Work out the finished part from the listing and answer in its coordinate system (mm). A direction names the side the tool comes from. Give positions to 0.01 mm unless a question says otherwise; leave off trailing zeros. Write each loop counter-clockwise with the first axis right and the second up, starting at its lowest first coordinate (ties: lowest second). Pieces come first, ordered by that corner, then holes.
1) Straight lines are drawn through the part: probe 1 along X at (y, z) = (0.95, 32); probe 2 along Z at (x, y) = (21.5, 0.85). For each, find the intervals that lie inside material, in ascending order.
2) Determine the mould class of faces 6 (the face through (-23, 2, -31)), 7 (the face through (-20, 2, -34)), 8 (the face through (25, 2, 0)) for opening direction X: pulls with the +X half, pulls with the -X half, needs draft (parallel to the pull), parting line crosses it, or undercut.
3) Given pin 1 Ø2.5 at (x, y) = (22, 3.5) entering from +Z; pin 2 Ø2.5 at (y, z) = (3, -32.5) entering from +X, each flat-ended and moving along its own axis, determine where each tip first touches the part or whether it passes through.
4) Find section A-A (y = 2.7). Determine the outline of the cut face in (x, z).
5) A tool of negligible diameter and unlimited length cuts with its end or side. For faces 1 (the face through (0, 2, -36)), 2 (the face through (22, 2, -31)), 3 (the face through (-22, 2, 31)), 4 (the face through (23, 2, 31)), 5 (the face through (0, 2, 36)), from which of +Z, -Z, +X, -X, +Y, -Y can it reach the whole face along a straight path? Write none if from no direction.
Autodesk Inventor part; units mm, degrees
ref_plane "YZ Plane" through (0, 0, 0) normal (1, 0, 0) x (0, 1, 0)
ref_plane "XZ Plane" through (0, 0, 0) normal (0, 1, 0) x (-1, 0, 0)
ref_plane "XY Plane" through (0, 0, 0) normal (0, 0, 1) x (1, 0, 0)
sketch "Sketch1" plane through (0, 0, 0) normal (0, 1, 0) x (-1, 0, 0)
  line L0 (25, -31) -> (-25, -31)
  line L1 (-25, -31) -> (-25, 31)
  line L2 (-25, 31) -> (25, 31)
  line L3 (25, 31) -> (25, -31)
  line L4 (25, -31) -> (-25, 31) construction
  line L5 (-25, -31) -> (25, 31) construction
  line L6 (-20, -36) -> (20, -36)
  line L7 (20, -36) -> (20, -31)
  line L8 (20, -31) -> (-20, -31)
  line L9 (-20, -31) -> (-20, -36)
  line L10 (-20, -36) -> (20, -31) construction
  line L11 (20, -36) -> (-20, -31) construction
  line L12 (-20, 31) -> (20, 31)
  line L13 (20, 31) -> (20, 36)
  line L14 (20, 36) -> (-20, 36)
  line L15 (-20, 36) -> (-20, 31)
  line L16 (-20, 31) -> (20, 36) construction
  line L17 (20, 31) -> (-20, 36) construction
  line L18 (0, 0) -> (0, -31) construction
  line L19 (0, -33.5) -> (0, -36) construction
  line L20 (0, 33.5) -> (0, 31) construction
  point P0 (-20, 31)
  point P1 (-20, -31)
  point P2 (20, -31)
  point P3 (20, 31)
  dimension "d0" = 5
  dimension "d1" = 5
  dimension "d2" = 40
  dimension "d3" = 40
  dimension "d4" = 62
  dimension "d5" = 50
extrude "Extrusion1" add sketch "Sketch1" along normal blind 5
properties part number "Base Plate Wall" material "PLA 33 Plastic"
Results:
1. probe 1: x = -20 to 20
1. probe 2: z = -31 to 31
2. face 6: needs draft
2. face 7: pulls with the -X half
2. face 8: pulls with the +X half
3. pin 1: stops at z = 31
3. pin 2: stops at x = 20
4. outline: (-25, -31) - (-20, -31) - (-20, -36) - (20, -36) - (20, -31) - (25, -31) - (25, 31) - (20, 31) - (20, 36) - (-20, 36) - (-20, 31) - (-25, 31) - close
5. face 1: -Z, +X, -X, +Y, -Y
5. face 2: -Z, +X, +Y, -Y
5. face 3: +Z, -X, +Y, -Y
5. face 4: +Z, +X, +Y, -Y
5. face 5: +Z, +X, -X, +Y, -Y
